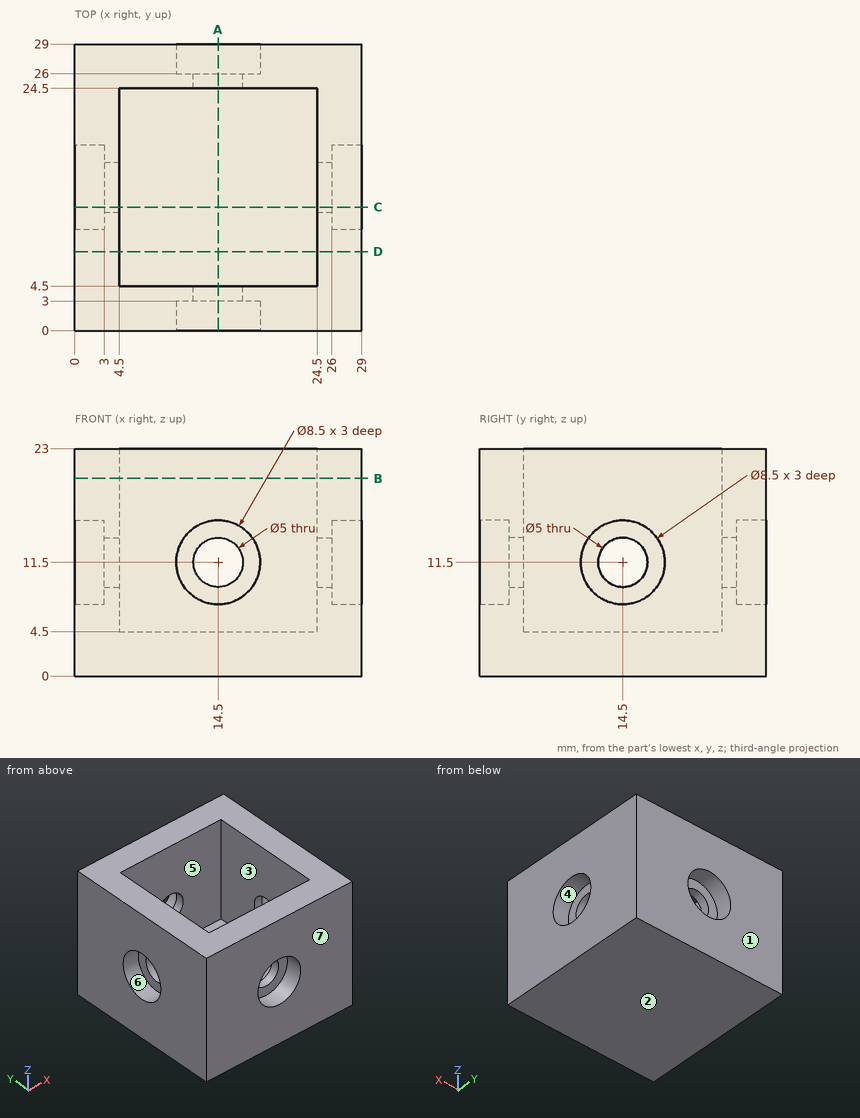
The drawing under review shows one solid part. Ordinate dimensions are in mm from its lowest x, y, z. A direction names the side the tool comes from. Round coordinates to 2 decimals unless told otherwise and drop trailing zeros. Order: outer loops, then holes, each group sorted by start corner. A loop starts at its lowest first (then second) coordinate and runs counter-clockwise, first axis right, second up. Notation, with made-up numbers: (-38, 2.5) -> (20, 2.5) arc R19 cw to (20, 17.5) -> close; hole circle Ø1 at (9.25, 30). An arc over 180 degrees is marked (long way). Return JSON: item names as keys, results as strings.
1. Take a section at B-B (z = 20). Write out the cut boundary in (x, y).
Answer block:
{"outline": "(0, 0) -> (29, 0) -> (29, 29) -> (0, 29) -> close; hole (4.5, 4.5) -> (24.5, 4.5) -> (24.5, 24.5) -> (4.5, 24.5) -> close"}
2. For L1, parallel to Z at x = 27.3, y = 14.5; L2, parallel to Y at x = 3.9, z = 11.5; L3, parallel to X at y = 18.5, z = 7.25, list the stretches that pass through material, from the lowest coordinate up. Write a range as [from, to].
Answer block:
{"L1": "z = [0, 7.25], [15.75, 23]", "L2": "y = [0, 12], [17, 29]", "L3": "x = [0, 4.5], [24.5, 29]"}
3. For the marked faces 5, 6 and 7, list the 3-axis set-ups (+Z, -Z, +X, -X, +Y, -Y) from which the entire face can be reached by the end or side of a thin tool; tool diameter is ignored.
Answer block:
{"face 5": "+Z", "face 6": "-X", "face 7": "+Z, -Z, +X, -X, -Y"}
4. Take a section at C-C (y = 12.5). Write out the cut boundary in (x, z).
Answer block:
{"outline": "(0, 0) -> (29, 0) -> (29, 7.75) -> (26, 7.75) -> (26, 10) -> (24.5, 10) -> (24.5, 4.5) -> (4.5, 4.5) -> (4.5, 10) -> (3, 10) -> (3, 7.75) -> (0, 7.75) -> close; (0, 15.25) -> (3, 15.25) -> (3, 13) -> (4.5, 13) -> (4.5, 23) -> (0, 23) -> close; (24.5, 13) -> (26, 13) -> (26, 15.25) -> (29, 15.25) -> (29, 23) -> (24.5, 23) -> close"}
5. Insertion check: P1, Ø5, axis at x = 6.5, z = 16.5, coming from the -Y side; P2, Ø5, axis at x = 14.5, y = 7.5, coming from the +Z side; P3, Ø4, axis at x = 14.5, z = 11.5, coming from the +Y side; P4, Ø6.5, axis at x = 14.5, z = 11.5, coming from the +Y side. Each pin has a flat end and moves straight along its axis. Give the tip position at first contact, or say it passes through.
Answer block:
{"P1": "stops at y = 0", "P2": "stops at z = 4.5", "P3": "passes through", "P4": "stops at y = 26"}
6. The part is to be moulded in two halves that separate along Y. For the marked faces 1, 2, 3 and 4, say which applies: +Y half, -Y half, draft (parallel to the pull), parting line (faces both ways), or undercut.
Answer block:
{"face 1": "+Y half", "face 2": "draft", "face 3": "undercut", "face 4": "undercut"}
7. Take a section at D-D (y = 8). Write out the cut boundary in (x, z), then the cut area to 3 significant figures.
Answer block:
{"outline": "(0, 0) -> (29, 0) -> (29, 23) -> (24.5, 23) -> (24.5, 4.5) -> (4.5, 4.5) -> (4.5, 23) -> (0, 23) -> close", "area": "297 mm²"}
8. Take a section at A-A (x = 14.5). Write out the cut boundary in (y, z).
Answer block:
{"outline": "(0, 0) -> (29, 0) -> (29, 7.25) -> (26, 7.25) -> (26, 9) -> (24.5, 9) -> (24.5, 4.5) -> (4.5, 4.5) -> (4.5, 9) -> (3, 9) -> (3, 7.25) -> (0, 7.25) -> close; (0, 15.75) -> (3, 15.75) -> (3, 14) -> (4.5, 14) -> (4.5, 23) -> (0, 23) -> close; (24.5, 14) -> (26, 14) -> (26, 15.75) -> (29, 15.75) -> (29, 23) -> (24.5, 23) -> close"}
